Could you check a few things on this model? Use its own coordinates, in mm. Face numbers are marked on the shaded views. Coordinates: 2 decimals unless noted, no trailing zeros. Loops run counter-clockwise (first coordinate to the right, second up) from the corner with the lowest first, then second, coordinate; pieces in that order, holes last. Notation, with made-up numbers: (70, 10.25) - (106, 10.25) arc R15 cw to (106, 15.25) - close; hole circle Ø7 at (-15, -23.5). An arc over 180 degrees is marked (long way). Use CSV: the item, a comma, the result in double quotes.
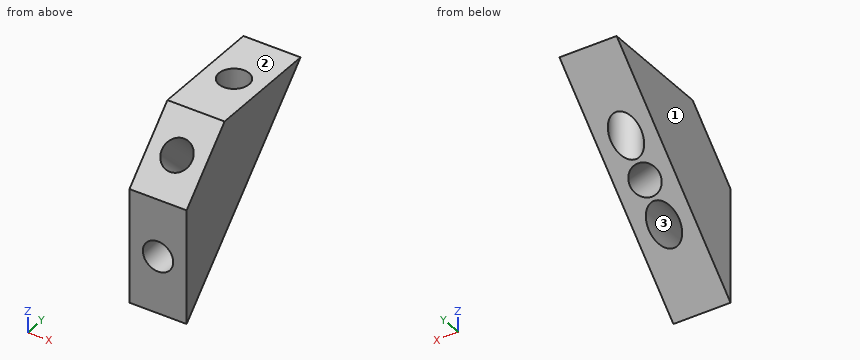
from build123d import *

# Parameters (mm, degrees)
PAD_DEPTH               = 5
SKETCH001_R             = 1.325
HOLE_DEPTH              = 15.0010000001
SKETCH002_R             = 1.325
HOLE001_DEPTH           = 17.6786695297
SKETCH003_R             = 1.325
HOLE002_DEPTH           = 15.001
BODY001_PLACEMENT_ANGLE = 90


with BuildPart() as part:
    # Sketch → Pad (new body)
    with BuildSketch(Plane.XZ.offset(-2.5)):
        Polygon((-10, 25.0000000001), (-19.9999999999, 25.0000000001), (-25, 20), (-25, 10), align=None)
    extrude(amount=PAD_DEPTH)

    # Sketch001 (on Face1 of Pad) → Hole (cut, through all)
    with BuildSketch(Plane(origin=(0, 0, 25.0000000001), x_dir=(-1, 0, 0), z_dir=(0, 0, 1))):
        with Locations((15, 0)):
            Circle(SKETCH001_R)
    extrude(amount=-HOLE_DEPTH, mode=Mode.SUBTRACT)

    # Sketch002 (on Face5 of Hole) → Hole001 (cut, through all)
    with BuildSketch(Plane(origin=(-22.5, 0, 22.5), x_dir=(-0.7071067812, 0, -0.7071067812), z_dir=(-0.7071067812, 0, 0.7071067812))):
        Circle(SKETCH002_R)
    extrude(amount=-HOLE001_DEPTH, mode=Mode.SUBTRACT)

    # Sketch003 (on Face7 of Hole001) → Hole002 (cut, through all)
    with BuildSketch(Plane(origin=(-25, 0, 0), x_dir=(0, 0, -1), z_dir=(-1, 0, 0))):
        with Locations((-15, 0)):
            Circle(SKETCH003_R)
    extrude(amount=-HOLE002_DEPTH, mode=Mode.SUBTRACT)


with BuildPart() as part_1:
    # Body001 placement: moved
    add(part.part.rotate(Axis((0, 0, 0), (0, 0, 1)), BODY001_PLACEMENT_ANGLE))


solid = part_1.part
(1) Please list where these lines run through material, in increasing order: line 1 (X direction, y = -21.5, z = 15) (3 decimals); line 2 (Z direction, x = 0.6, y = -17); line 3 (Y direction, x = 0.15, z = 19.75).
Computed:
line 1,"x = -2.5 to -1.325, 1.325 to 2.5"
line 2,"z = 18.67 to 25"
line 3,"y = -25 to -21.61, -17.89 to -16.32"
(2) Suppose I cut it at B-B (z = 15). Write out the boundary of the cut face in (x, y) (3 decimals).
Computed:
outline,"(-2.5, -25) - (-1.325, -25) - (-1.325, -20) - (-2.5, -20) - close; (1.325, -25) - (2.5, -25) - (2.5, -20) - (1.325, -20) - close"
(3) Thinking about a two-plate mould opening in X: for the marked faces 1, 2 and 3, which applies, +X half, -X half, draft (parallel to the pull), parting line (faces both ways), or undercut?
Computed:
face 1,"-X half"
face 2,"draft"
face 3,"undercut"
(4) Suppose I cut it at C-C (x = -0.75). Write out the boundary of the cut face in (y, z).
Computed:
outline,"(-25, 10) - (-21.09, 13.91) - (-25, 13.91) - close; (-25, 16.09) - (-18.91, 16.09) - (-18.27, 16.73) - (-23.27, 21.73) - (-25, 20) - close; (-21.73, 23.27) - (-16.73, 18.27) - (-16.09, 18.91) - (-16.09, 25) - (-20, 25) - close; (-13.91, 21.09) - (-10, 25) - (-13.91, 25) - close"
(5) Suppose I cut it at A-A (y = -15). Write out the boundary of the cut face in (x, z) (3 decimals).
Computed:
outline,"(-2.5, 20) - (-1.325, 20) - (-1.325, 25) - (-2.5, 25) - close; (1.325, 20) - (2.5, 20) - (2.5, 25) - (1.325, 25) - close"
(6) Will this pin go through, and if not, where does the flat tip stop? pin 1 (1 mm diameter, centred on x = 0, z = 19.5, fed in from +Y).
Computed:
pin 1,"stops at y = -16.23"
(7) Suppose I cut it at D-D (z = 24). Write out the boundary of the cut face in (x, y) (3 decimals), plus the area to 3 significant figures.
Computed:
outline,"(-2.5, -21) - (2.5, -21) - (2.5, -11) - (-2.5, -11) - close; hole circle Ø2.65 at (0, -15)"
area,"44.5 mm²"
